Source: CAD feature listing. Evaluate the final solid. Frame: model axes, mm. A direction names the side the tool comes from. Round coordinates to 2 decimals unless told otherwise and drop trailing zeros. Write each loop counter-clockwise with the first axis right and the second up, starting at its lowest first coordinate (ties: lowest second). Pieces come first, ordered by that corner, then holes.
from build123d import *

# Parameters (mm, degrees)
F0_W      = 2438.4
F0_H      = 1219.2
F1_DEPTH  = 25.4
F2_W      = 2438.4
F2_H      = 1219.2
F2_W_2    = 2362.2
F2_H_2    = 1143
F3_DEPTH  = 88.9
F4_W      = 38.1
F4_H      = 88.9
F5_DEPTH  = 895.35
F7_W      = 1104.9
F7_H      = 1143
F7_W_2    = 1066.8
F8_DEPTH  = 88.9
F9_W      = 2286
F9_H      = 1219.2
F10_DEPTH = 12.7


with BuildPart() as f1:
    # F0 (on Top) → F1 (new body)
    with BuildSketch(Plane.XY):
        with Locations((1219.2, -609.6)):
            Rectangle(F0_W, F0_H)
    extrude(amount=F1_DEPTH)

    # F2 (on face) → F3 (join)
    with BuildSketch(Plane(origin=(0, 0, 0), x_dir=(1, 0, 0), z_dir=(0, 0, -1))):
        with Locations((1219.2, 609.6)):
            Rectangle(F2_W, F2_H)
        with Locations((1219.2, 609.6)):
            Rectangle(F2_W_2, F2_H_2, mode=Mode.SUBTRACT)
    extrude(amount=F3_DEPTH)

    # F4 (on face) → F5 (join)
    with BuildSketch(Plane(origin=(0, 0, 0), x_dir=(1, 0, 0), z_dir=(0, 0, -1))):
        with Locations((57.15, 1136.65)):
            Rectangle(F4_W, F4_H)
        with Locations((57.15, 82.55)):
            Rectangle(F4_W, F4_H)
        with Locations((2381.25, 1136.65)):
            Rectangle(F4_W, F4_H)
        with Locations((2381.25, 82.55)):
            Rectangle(F4_W, F4_H)
        with Locations((1200.15, 1136.65)):
            Rectangle(F4_W, F4_H)
        with Locations((1200.15, 82.55)):
            Rectangle(F4_W, F4_H)
    extrude(amount=F5_DEPTH)

    # F7 (on offset) → F8 (join)
    with BuildSketch(Plane.XY.offset(-730.25)):
        Polygon((2400.3, 0), (38.1, 0), (38.1, -38.1), (76.2, -38.1), (76.2, -1181.1), (38.1, -1181.1), (38.1, -1219.2), (2400.3, -1219.2), (2400.3, -1181.1), (2362.2, -1181.1), (2362.2, -38.1), (2400.3, -38.1), align=None)
        with Locations((666.75, -609.6)):
            Rectangle(F7_W, F7_H, mode=Mode.SUBTRACT)
        with Locations((1790.7, -609.6)):
            Rectangle(F7_W_2, F7_H, mode=Mode.SUBTRACT)
    extrude(amount=-F8_DEPTH)

    # F9 (on offset) → F10 (join)
    with BuildSketch(Plane.XY.offset(-730.25)):
        with Locations((1219.2, -609.6)):
            Rectangle(F9_W, F9_H)
    extrude(amount=F10_DEPTH)


solid = f1.part
1) Section query A-A on x = 1111. Return the cut outline in (y, z).
Taken from the geometry:
outline: (-1219.2, -819.15) - (-1181.1, -819.15) - (-1181.1, -730.25) - (-38.1, -730.25) - (-38.1, -819.15) - (0, -819.15) - (0, -717.55) - (-1219.2, -717.55) - close; (-1219.2, -88.9) - (-1181.1, -88.9) - (-1181.1, 0) - (-38.1, 0) - (-38.1, -88.9) - (0, -88.9) - (0, 25.4) - (-1219.2, 25.4) - close
2) Section query B-B on y = -320.5. Return the cut outline in (x, z), then the cut area to 3 significant figures.
Taken from the geometry:
outline: (0, -88.9) - (38.1, -88.9) - (38.1, 0) - (2400.3, 0) - (2400.3, -88.9) - (2438.4, -88.9) - (2438.4, 25.4) - (0, 25.4) - close; (76.2, -819.15) - (114.3, -819.15) - (114.3, -730.25) - (1219.2, -730.25) - (1219.2, -819.15) - (1257.3, -819.15) - (1257.3, -730.25) - (2324.1, -730.25) - (2324.1, -819.15) - (2362.2, -819.15) - (2362.2, -717.55) - (76.2, -717.55) - close
area: 108,000 mm2
3) Section query C-C on z = -431.5. Return the cut outline in (x, y), then the cut area to 3 significant figures.
Taken from the geometry:
outline: (38.1, -1181.1) - (76.2, -1181.1) - (76.2, -1092.2) - (38.1, -1092.2) - close; (38.1, -127) - (76.2, -127) - (76.2, -38.1) - (38.1, -38.1) - close; (1181.1, -1181.1) - (1219.2, -1181.1) - (1219.2, -1092.2) - (1181.1, -1092.2) - close; (1181.1, -127) - (1219.2, -127) - (1219.2, -38.1) - (1181.1, -38.1) - close; (2362.2, -1181.1) - (2400.3, -1181.1) - (2400.3, -1092.2) - (2362.2, -1092.2) - close; (2362.2, -127) - (2400.3, -127) - (2400.3, -38.1) - (2362.2, -38.1) - close
area: 20,300 mm2
4) Reachability of faces 3 (the face through (1783, -1181.1, -44)), 4 (the face through (38.1, -603, -44)), 5 (the face through (2362.2, -1136, -857)), 6 (the face through (2400.3, -1142, -486)), 7 (the face through (2362.2, -616, -769)) from +Z, -Z, +X, -X, +Y, -Y: full face, straight path, thin tool, end or side. Return the list, or none.
Taken from the geometry:
face 3: none
face 4: -Z
face 5: -Z, +Y, -Y
face 6: -Z, +X, +Y, -Y
face 7: -Z, +X
5) Contact query for flat-ended pins moving along their axis: P1, Ø6.5, axis at y = -20, z = -723, coming from the -X side; P2, Ø11.5, axis at x = 2382.5, z = -464.5, coming from the +Y side; P3, Ø10, axis at y = -17.5, z = -723, coming from the +X side. Output: stop coordinate, or through.
Taken from the geometry:
P1: stops at x = 76.2
P2: stops at y = -38.1
P3: stops at x = 2362.2
6) Material intervals for line 1 (X direction, y = -1034.5, z = -780); line 2 (X direction, y = -1139.5, z = -169.5); line 3 (Y direction, x = 1798.5, z = -72.5), sorted ascending.
Taken from the geometry:
line 1: x = 76.2 to 114.3, 1219.2 to 1257.3, 2324.1 to 2362.2
line 2: x = 38.1 to 76.2, 1181.1 to 1219.2, 2362.2 to 2400.3
line 3: y = -1219.2 to -1181.1, -38.1 to 0
7) Pull-direction query (Z, two-part tool) for faces 1 (the face through (76.2, -82, -354)), 2 (the face through (640, -38.1, -774)); classes: released by +Z, released by -Z, zero draft, split by the parting line, or undercut.
Taken from the geometry:
face 1: undercut
face 2: zero draft
8) Section query D-D on z = -48.5. Return the cut outline in (x, y).
Taken from the geometry:
outline: (0, -1219.2) - (2438.4, -1219.2) - (2438.4, 0) - (0, 0) - close; hole (38.1, -1092.2) - (76.2, -1092.2) - (76.2, -1181.1) - (1181.1, -1181.1) - (1181.1, -1092.2) - (1219.2, -1092.2) - (1219.2, -1181.1) - (2362.2, -1181.1) - (2362.2, -1092.2) - (2400.3, -1092.2) - (2400.3, -127) - (2362.2, -127) - (2362.2, -38.1) - (1219.2, -38.1) - (1219.2, -127) - (1181.1, -127) - (1181.1, -38.1) - (76.2, -38.1) - (76.2, -127) - (38.1, -127) - close
